The model under review builds one solid part; all positions refer to its coordinate system, in mm. A direction names the side the tool comes from. Give positions to 0.01 mm unless a question says otherwise; leave off trailing zeros. Order: outer loops, then holes, each group sorted by start corner. A loop starts at its lowest first (then second) coordinate and runs counter-clockwise, first axis right, second up.
```python
from build123d import *

# Parameters (mm, degrees)
PAD_DEPTH           = 710
HOLE_D              = 3.4
HOLE_DEPTH          = 25
HOLE_CBORE_D        = 5.8
HOLE_CBORE_DEPTH    = 1.5
HOLE_TIPS_R         = 1.7
HOLE001_D           = 3.4
HOLE001_DEPTH       = 25
HOLE001_CBORE_D     = 5.5
HOLE001_CBORE_DEPTH = 1.5
HOLE001_TIPS_R      = 1.7
SKETCH004_R         = 7
POCKET_DEPTH        = 3
SKETCH005_R         = 1.7
HOLE002_DEPTH       = 25
HOLE002_TIPS_R      = 1.7
POCKET001_DEPTH     = 47.001
SKETCH007_R         = 1.7
HOLE003_DEPTH       = 25
HOLE003_TIPS_R      = 1.7
SKETCH009_R         = 12
POCKET002_DEPTH     = 12.501
SKETCH011_R         = 1.7
HOLE004_DEPTH       = 50.001
SKETCH010_R         = 1.7
HOLE005_DEPTH       = 50.001
SKETCH012_R         = 7
POCKET003_DEPTH     = 3
POCKET004_DEPTH     = 47.001
SKETCH014_R         = 1.7
HOLE006_DEPTH       = 25
HOLE006_TIPS_R      = 1.7


with BuildPart() as part:
    # Sketch → Pad (new body)
    with BuildSketch(Plane.XZ):
        Polygon((0, 0), (-44, 0), (-44, 8.5), (-5.5, 8.5), (-5.5, 50), (7, 50), (7, 45), (0, 45), align=None)
    extrude(amount=PAD_DEPTH)

    # Hole
    with Locations(Plane(origin=(0, 0, 50), x_dir=(-1, 0, 0), z_dir=(0, 0, 1))):
        with Locations((-3.5, 85), (-3.5, 635)):
            CounterBoreHole(HOLE_D / 2, HOLE_CBORE_D / 2, HOLE_CBORE_DEPTH, depth=HOLE_DEPTH)

    # Hole tips → Hole tip 1 section 0
    with BuildSketch(Plane(origin=(0, 0, 25), x_dir=(-1, 0, 0), z_dir=(0, 0, 1)), mode=Mode.PRIVATE) as hole_tip_1_s0:
        with Locations((-3.5, 85)):
            Circle(HOLE_TIPS_R)
    loft([hole_tip_1_s0.sketch, Vertex(3.5, -85, 23.978537)], mode=Mode.SUBTRACT)

    # Hole tips → Hole tip 2 section 0
    with BuildSketch(Plane(origin=(0, 0, 25), x_dir=(-1, 0, 0), z_dir=(0, 0, 1)), mode=Mode.PRIVATE) as hole_tip_2_s0:
        with Locations((-3.5, 635)):
            Circle(HOLE_TIPS_R)
    loft([hole_tip_2_s0.sketch, Vertex(3.5, -635, 23.978537)], mode=Mode.SUBTRACT)

    # Hole001
    with Locations(Plane(origin=(0, 0, 50), x_dir=(-1, 0, 0), z_dir=(0, 0, 1))):
        with Locations((-3.5, 375)):
            CounterBoreHole(HOLE001_D / 2, HOLE001_CBORE_D / 2, HOLE001_CBORE_DEPTH, depth=HOLE001_DEPTH)

    # Hole001 tips → Hole001 tip 1 section 0
    with BuildSketch(Plane(origin=(0, 0, 25), x_dir=(-1, 0, 0), z_dir=(0, 0, 1)), mode=Mode.PRIVATE) as hole001_tip_1_s0:
        with Locations((-3.5, 375)):
            Circle(HOLE001_TIPS_R)
    loft([hole001_tip_1_s0.sketch, Vertex(3.5, -375, 23.978537)], mode=Mode.SUBTRACT)

    # Sketch004 → Pocket (cut)
    with BuildSketch(Plane(origin=(0, 0, 0), x_dir=(1, 0, 0), z_dir=(0, 0, -1))):
        with Locations((-20.75, 55)):
            Circle(SKETCH004_R)
    extrude(amount=-POCKET_DEPTH, mode=Mode.SUBTRACT)

    # Sketch005 (on Face1 of Pocket) → Hole002 (cut)
    with BuildSketch(Plane(origin=(0, 0, 0), x_dir=(1, 0, 0), z_dir=(0, 0, -1))):
        with Locations((-31.5, 55)):
            Circle(SKETCH005_R)
        with Locations((-9.5, 55)):
            Circle(SKETCH005_R)
    extrude(amount=-HOLE002_DEPTH, mode=Mode.SUBTRACT)

    # Hole002 tips → Hole002 tip 1 section 0
    with BuildSketch(Plane(origin=(0, 0, 25), x_dir=(1, 0, 0), z_dir=(0, 0, -1)), mode=Mode.PRIVATE) as hole002_tip_1_s0:
        with Locations((-31.5, 55)):
            Circle(HOLE002_TIPS_R)
    loft([hole002_tip_1_s0.sketch, Vertex(-31.5, -55, 26.021463)], mode=Mode.SUBTRACT)

    # Hole002 tips → Hole002 tip 2 section 0
    with BuildSketch(Plane(origin=(0, 0, 25), x_dir=(1, 0, 0), z_dir=(0, 0, -1)), mode=Mode.PRIVATE) as hole002_tip_2_s0:
        with Locations((-9.5, 55)):
            Circle(HOLE002_TIPS_R)
    loft([hole002_tip_2_s0.sketch, Vertex(-9.5, -55, 26.021463)], mode=Mode.SUBTRACT)

    # Sketch006 → Pocket001 (cut, through all)
    with BuildSketch(Plane(origin=(0, 0, 3), x_dir=(1, 0, 0), z_dir=(0, 0, -1))):
        with BuildLine():
            ThreePointArc((-23.25, 56.2), (-24.45, 55), (-23.25, 53.8))
            Line((-23.25, 53.8), (-18.25, 53.8))
            ThreePointArc((-18.25, 53.8), (-17.05, 55), (-18.25, 56.2))
            Line((-18.25, 56.2), (-23.25, 56.2))
        make_face()
    extrude(amount=-POCKET001_DEPTH, mode=Mode.SUBTRACT)

    # Sketch007 → Hole003 (cut)
    with BuildSketch(Plane(origin=(0, 0, 3), x_dir=(1, 0, 0), z_dir=(0, 0, -1))):
        with Locations((-23.25, 55)):
            Circle(SKETCH007_R)
        with Locations((-18.25, 55)):
            Circle(SKETCH007_R)
    extrude(amount=-HOLE003_DEPTH, mode=Mode.SUBTRACT)

    # Hole003 tips → Hole003 tip 1 section 0
    with BuildSketch(Plane(origin=(0, 0, 28), x_dir=(1, 0, 0), z_dir=(0, 0, -1)), mode=Mode.PRIVATE) as hole003_tip_1_s0:
        with Locations((-23.25, 55)):
            Circle(HOLE003_TIPS_R)
    loft([hole003_tip_1_s0.sketch, Vertex(-23.25, -55, 29.021463)], mode=Mode.SUBTRACT)

    # Hole003 tips → Hole003 tip 2 section 0
    with BuildSketch(Plane(origin=(0, 0, 28), x_dir=(1, 0, 0), z_dir=(0, 0, -1)), mode=Mode.PRIVATE) as hole003_tip_2_s0:
        with Locations((-18.25, 55)):
            Circle(HOLE003_TIPS_R)
    loft([hole003_tip_2_s0.sketch, Vertex(-18.25, -55, 29.021463)], mode=Mode.SUBTRACT)

    # Sketch009 → Pocket002 (cut, through all)
    with BuildSketch(Plane(origin=(-5.5, 0, 0), x_dir=(0, 0, -1), z_dir=(-1, 0, 0))):
        with Locations((-29.25, 55)):
            Circle(SKETCH009_R)
    extrude(amount=-POCKET002_DEPTH, mode=Mode.SUBTRACT)

    # Sketch011 → Hole004 (cut, through all)
    with BuildSketch(Plane(origin=(0, 0, 0), x_dir=(1, 0, 0), z_dir=(0, 0, -1))):
        with Locations((-20.75, 690)):
            Circle(SKETCH011_R)
        with Locations((-20.75, 680)):
            Circle(SKETCH011_R)
    extrude(amount=-HOLE004_DEPTH, mode=Mode.SUBTRACT)

    # Sketch010 → Hole005 (cut, through all)
    with BuildSketch(Plane(origin=(0, 0, 0), x_dir=(1, 0, 0), z_dir=(0, 0, -1))):
        with Locations((-31.125, 575)):
            Circle(SKETCH010_R)
        with Locations((-10.375, 575)):
            Circle(SKETCH010_R)
    extrude(amount=-HOLE005_DEPTH, mode=Mode.SUBTRACT)

    # Sketch012 → Pocket003 (cut)
    with BuildSketch(Plane(origin=(0, 0, 0), x_dir=(1, 0, 0), z_dir=(0, 0, -1))):
        with Locations((-20.75, 575)):
            Circle(SKETCH012_R)
    extrude(amount=-POCKET003_DEPTH, mode=Mode.SUBTRACT)

    # Sketch013 → Pocket004 (cut, through all)
    with BuildSketch(Plane(origin=(0, 0, 3), x_dir=(1, 0, 0), z_dir=(0, 0, -1))):
        with BuildLine():
            ThreePointArc((-23.25, 576.2), (-24.45, 575), (-23.25, 573.8))
            Line((-23.25, 573.8), (-18.25, 573.8))
            ThreePointArc((-18.25, 573.8), (-17.05, 575), (-18.25, 576.2))
            Line((-18.25, 576.2), (-23.25, 576.2))
        make_face()
    extrude(amount=-POCKET004_DEPTH, mode=Mode.SUBTRACT)

    # Sketch014 → Hole006 (cut)
    with BuildSketch(Plane(origin=(0, 0, 3), x_dir=(1, 0, 0), z_dir=(0, 0, -1))):
        with Locations((-18.25, 575)):
            Circle(SKETCH014_R)
        with Locations((-23.25, 575)):
            Circle(SKETCH014_R)
    extrude(amount=-HOLE006_DEPTH, mode=Mode.SUBTRACT)

    # Hole006 tips → Hole006 tip 1 section 0
    with BuildSketch(Plane(origin=(0, 0, 28), x_dir=(1, 0, 0), z_dir=(0, 0, -1)), mode=Mode.PRIVATE) as hole006_tip_1_s0:
        with Locations((-18.25, 575)):
            Circle(HOLE006_TIPS_R)
    loft([hole006_tip_1_s0.sketch, Vertex(-18.25, -575, 29.021463)], mode=Mode.SUBTRACT)

    # Hole006 tips → Hole006 tip 2 section 0
    with BuildSketch(Plane(origin=(0, 0, 28), x_dir=(1, 0, 0), z_dir=(0, 0, -1)), mode=Mode.PRIVATE) as hole006_tip_2_s0:
        with Locations((-23.25, 575)):
            Circle(HOLE006_TIPS_R)
    loft([hole006_tip_2_s0.sketch, Vertex(-23.25, -575, 29.021463)], mode=Mode.SUBTRACT)


solid = part.part
```
1. Take a section at A-A (z = 29.25). Write out the cut boundary in (x, y), and give its area (3 significant figures).
2. Draft analysis for pull direction Z (two halves, no side actions). For faces 1 (the flat face through (1, -350, 50)), 2 (the cylindrical face through (-2.788, -44.354, 23.713)), 3 (the flat face through (-13, -710, 8)), 4 (the flat face through (-22, -350, 0)), state which applies: pulls with the +Z half, pulls with the -Z half, needs draft (parallel to the pull), parting line crosses it, or undercut.
3. Insertion check: pin 1 (4 mm diameter, centred on y = -304, z = 11, fed in from +X); pin 2 (4 mm diameter, centred on x = 3.5, y = -375, fed in from +Z); pin 3 (11 mm diameter, centred on x = -21, y = -54, fed in from -Z). Each pin has a flat end and moves straight along its axis. Give the tip position at first contact, or say it passes through.
4. To check wall thickness, follow line 1 (X direction, y = -55, z = 1.65); line 2 (Y direction, x = 3.5, z = 48.9); line 3 (Y direction, x = -18.25, z = 7.35). State the ranges of each line that lie inside material, in increasing order.
5. Take a section at B-B (y = -611). Write out the cut boundary in (x, z), and give its area (3 significant figures).
6. For faces 5 (the flat face through (-25, -350, 8.5)), 6 (the flat face through (-13, 0, 8)), 7 (the flat face through (0, -350, 23)), 8 (the flat face through (-20.8, -53.5, 3)), list the 3-axis set-ups (+Z, -Z, +X, -X, +Y, -Y) from which the entire face can be reached by the end or side of a thin tool; tool diameter is ignored.
Answer:
1. outline: (-5.5, -710) - (0, -710) - (0, -67) - (-5.5, -67) - close; (-5.5, -43) - (0, -43) - (0, 0) - (-5.5, 0) - close
1. area: 3,770 mm2
2. face 1: pulls with the +Z half
2. face 2: undercut
2. face 3: needs draft
2. face 4: pulls with the -Z half
3. pin 1: stops at x = 0
3. pin 2: stops at z = 48.5
3. pin 3: stops at z = 3
4. line 1: x = -44 to -33.2, -29.8 to -27.75, -13.75 to -11.2, -7.8 to 0
4. line 2: y = -710 to -637.9, -632.1 to -377.75, -372.25 to -87.9, -82.1 to 0
4. line 3: y = -710 to -576.7, -573.3 to -56.7, -53.3 to 0
5. outline: (-44, 0) - (0, 0) - (0, 45) - (7, 45) - (7, 50) - (-5.5, 50) - (-5.5, 8.5) - (-44, 8.5) - close
5. area: 637 mm2
6. face 5: +Z, -X, +Y, -Y
6. face 6: +Z, -Z, +X, -X, +Y
6. face 7: -Z, +X, +Y, -Y
6. face 8: -Z
